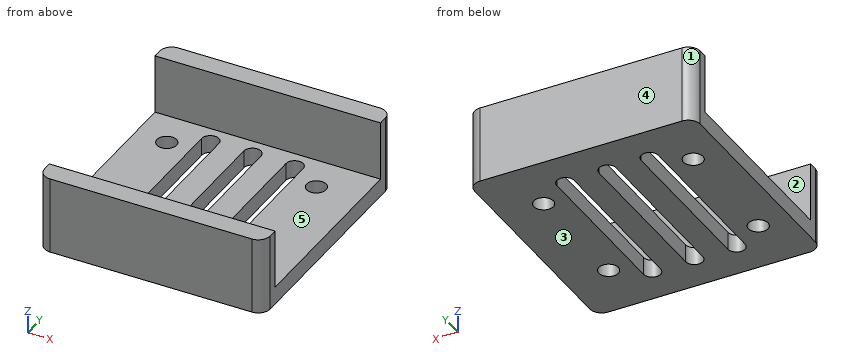
from build123d import *

# Parameters (mm, degrees)
SKETCH1_R           = 1.65
BOSS_EXTRUDE1_DEPTH = 13
CUT_EXTRUDE1_DEPTH  = 32.128764833
SKETCH3_W           = 52.718311268
SKETCH3_H           = 33
CUT_EXTRUDE2_DEPTH  = 10


with BuildPart() as part:
    # Sketch1 → Boss-Extrude1 (new body)
    with BuildSketch(Plane.XY):
        with BuildLine():
            Line((0, 20), (-16, 20))
            ThreePointArc((-16, 20), (-17.414213562, 19.414213562), (-18, 18))
            Line((-18, 18), (-18, -18))
            ThreePointArc((-18, -18), (-17.414213562, -19.414213562), (-16, -20))
            Line((-16, -20), (0, -20))
            Line((0, -20), (18, -20))
            ThreePointArc((18, -20), (19.414213562, -19.414213562), (20, -18))
            Line((20, -18), (20, 18))
            ThreePointArc((20, 18), (19.414213562, 19.414213562), (18, 20))
            Line((18, 20), (0, 20))
        make_face()
        with Locations(Location((-12.6, 10.16, 0), (0, 0, 180))):
            Circle(SKETCH1_R, mode=Mode.SUBTRACT)
        with Locations(Location((12.6, 10.16, 0), (0, 0, 180))):
            Circle(SKETCH1_R, mode=Mode.SUBTRACT)
        with Locations(Location((12.6, -10.16, 0), (0, 0, 180))):
            Circle(SKETCH1_R, mode=Mode.SUBTRACT)
        with Locations(Location((-12.6, -10.16, 0), (0, 0, 180))):
            Circle(SKETCH1_R, mode=Mode.SUBTRACT)
    extrude(amount=BOSS_EXTRUDE1_DEPTH)

    # Sketch2 → Cut-Extrude1 (cut, through all)
    with BuildSketch(Plane.XY.offset(13)):
        with BuildLine():
            Line((5.65, -13.55), (5.65, 13.55))
            ThreePointArc((5.65, 13.55), (7.1, 15), (8.55, 13.55))
            Line((8.55, 13.55), (8.55, -13.55))
            ThreePointArc((8.55, -13.55), (7.1, -15), (5.65, -13.55))
        make_face()
        with BuildLine():
            Line((1.45, -13.55), (1.45, 13.55))
            ThreePointArc((1.45, 13.55), (0, 15), (-1.45, 13.55))
            Line((-1.45, 13.55), (-1.45, -13.55))
            ThreePointArc((-1.45, -13.55), (0, -15), (1.45, -13.55))
        make_face()
        with BuildLine():
            Line((-8.55, -13.55), (-8.55, 13.55))
            ThreePointArc((-8.55, 13.55), (-7.1, 15), (-5.65, 13.55))
            Line((-5.65, 13.55), (-5.65, -13.55))
            ThreePointArc((-5.65, -13.55), (-7.1, -15), (-8.55, -13.55))
        make_face()
    extrude(amount=-CUT_EXTRUDE1_DEPTH, mode=Mode.SUBTRACT)

    # Sketch3 → Cut-Extrude2 (cut)
    with BuildSketch(Plane.XY.offset(13)):
        Rectangle(SKETCH3_W, SKETCH3_H)
    extrude(amount=-CUT_EXTRUDE2_DEPTH, mode=Mode.SUBTRACT)


solid = part.part
Design review of the part built by this model. Coordinates are the model's own, in mm. Face numbers are marked on the shaded views. A direction names the side the tool comes from. Coordinates: 2 decimals unless noted, no trailing zeros. Order: outer loops, then holes, each group sorted by start corner. A loop starts at its lowest first (then second) coordinate and runs counter-clockwise, first axis right, second up. Notation, with made-up numbers: (-27, -28.5) - (-12, -28.5) arc R12 cw to (-12, -20.5) - close; hole circle Ø3 at (-26.5, -19). An arc over 180 degrees is marked (long way). Put each result on its own line as item: value.
1) The part is to be moulded in two halves that separate along Y. For the marked faces 3, 4 and 5, say which applies: released by +Y, released by -Y, zero draft, split by the parting line, or undercut.
Response values:
face 3: zero draft
face 4: released by +Y
face 5: undercut
2) Tool access review of the marked faces 1 and 2: name each direction out of +Z, -Z, +X, -X, +Y, -Y from which nothing blocks a thin tool from reaching the whole face with its end or side.
Response values:
face 1: +Z, -Z, -X, +Y
face 2: +Z, +X, -X
3) Take a section at B-B, the plane z = 10.25. Give the boundary of the cut face in (x, y), and give its area (3 significant figures).
Response values:
outline: (-18, -18) arc R2 ccw to (-16, -20) - (18, -20) arc R2 ccw to (20, -18) - (20, -16.5) - (-18, -16.5) - close; (-18, 16.5) - (20, 16.5) - (20, 18) arc R2 ccw to (18, 20) - (-16, 20) arc R2 ccw to (-18, 18) - close
area: 263 mm²
4) Take a section at D-D, the plane x = 7.1. Give the boundary of the cut face in (y, z), and give its area (3 significant figures).
Response values:
outline: (-20, 0) - (-15, 0) - (-15, 3) - (-16.5, 3) - (-16.5, 13) - (-20, 13) - close; (15, 0) - (20, 0) - (20, 13) - (16.5, 13) - (16.5, 3) - (15, 3) - close
area: 100 mm²
5) Insertion check: P1, Ø2, axis at x = 12, y = -10.5, coming from the -Z side; P2, Ø16.5, axis at x = 6.5, y = 7.5, coming from the +Z side. Each pin has a flat end and moves straight along its axis. Give the tip position at first contact, or say it passes through.
Response values:
P1: stops at z = 0
P2: stops at z = 3
6) Take a section at A-A, the plane y = 4. Give the boundary of the cut face in (x, z).
Response values:
outline: (-18, 0) - (-8.55, 0) - (-8.55, 3) - (-18, 3) - close; (-5.65, 0) - (-1.45, 0) - (-1.45, 3) - (-5.65, 3) - close; (1.45, 0) - (5.65, 0) - (5.65, 3) - (1.45, 3) - close; (8.55, 0) - (20, 0) - (20, 3) - (8.55, 3) - close
7) Wall thickness on L1, parallel to Y at x = 12.6, z = 1.5; L2, parallel to X at y = 13.5, z = 2.75; L3, parallel to X at y = 10.16, z = 2.1: over which ranges is each line inside the solid? List them lowest first. Write a range as from..to.
Response values:
L1: y = -20..-11.81, -8.51..8.51, 11.81..20
L2: x = -18..-8.55, -5.65..-1.45, 1.45..5.65, 8.55..20
L3: x = -18..-14.25, -10.95..-8.55, -5.65..-1.45, 1.45..5.65, 8.55..10.95, 14.25..20
8) Take a section at C-C, the plane x = 12.6. Give the boundary of the cut face in (y, z), and give its area (3 significant figures).
Response values:
outline: (-20, 0) - (-11.81, 0) - (-11.81, 3) - (-16.5, 3) - (-16.5, 13) - (-20, 13) - close; (-8.51, 0) - (8.51, 0) - (8.51, 3) - (-8.51, 3) - close; (11.81, 0) - (20, 0) - (20, 13) - (16.5, 13) - (16.5, 3) - (11.81, 3) - close
area: 170 mm²
